Can you work these out from the model? Positions are in its coordinate system, mm. Coordinates: 2 decimals unless noted, no trailing zeros. Order: outer loops, then holes, each group sorted by start corner. A loop starts at its lowest first (then second) coordinate and runs counter-clockwise, first axis right, second up. Notation, with made-up numbers: (-11, 42.25) -> (36, 42.25) arc R28 ccw to (36, 70.25) -> close; hole circle Ø4 at (64.25, 44.25). An arc over 180 degrees is marked (long way). Return JSON: item names as keys, results as strings. Group by question number.
1) If I drill on probe 1 along Y at (x, z) = (62.5, 2.65); probe 2 along Y at (x, z) = (88.5, 0.95); probe 3 along Y at (x, z) = (99, 0.7), over which ranges is the centre line in solid material (lowest first)? Write a range as from..to.
2) If we section it at B-B, the plane y = 3755: Please give me the cut outline in (x, z), then the cut area to 3 significant figures.
3) If we section it at A-A, the plane z = 1.35: Please give me the cut outline in (x, y), then the cut area to 3 significant figures.
4) For pin 1 (11 mm diameter, centred on x = 106.6, y = 3258.06, fed in from -Z); pin 2 (23.5 mm diameter, centred on x = 86.75, y = 4138.87, fed in from -Z), each with a flat end and sliding along its axis, tell me the tip position at first contact or that it passes through.
Autodesk Inventor part; units mm, degrees
ref_plane "YZ Plane" through (0, 0, 0) normal (1, 0, 0) x (0, 1, 0)
ref_plane "XZ Plane" through (0, 0, 0) normal (0, 1, 0) x (-1, 0, 0)
ref_plane "XY Plane" through (0, 0, 0) normal (0, 0, 1) x (1, 0, 0)
sketch "Sketch1" plane through (0, 0, 0) normal (0, 0, 1) x (1, 0, 0)
  line L0 (0, 0) -> (0, 4438.8737)
  line L1 (0, 4438.8737) -> (100, 4438.8737)
  line L2 (100, 4438.8737) -> (200, 0)
  line L3 (200, 0) -> (0, 0)
  circle A0 centre (0, 0) radius 30
  line L4 (0, 1479.6246) -> (166.6667, 1479.6246)
  line L5 (0, 2959.2492) -> (133.3333, 2959.2492)
  circle A1 centre (0, 1479.6246) radius 30
  circle A2 centre (0, 2959.2492) radius 30
  line L6 (190.8761, 405) -> (120.8761, 405)
  line L7 (120.8761, 405) -> (120.8761, 410)
  line L8 (120.8761, 410) -> (190.8761, 410)
  line L9 (190.8761, 410) -> (190.8761, 405)
  line L10 (109.6148, 909.8732) -> (179.6148, 909.8732)
  line L11 (179.6148, 904.8732) -> (109.6148, 904.8732)
  line L12 (109.6148, 904.8732) -> (109.6148, 909.8732)
  line L13 (179.6148, 909.8732) -> (179.6148, 904.8732)
  line L14 (98.3535, 1409.7463) -> (168.3535, 1409.7463)
  line L15 (168.3535, 1404.7463) -> (98.3535, 1404.7463)
  line L16 (98.3535, 1404.7463) -> (98.3535, 1409.7463)
  line L17 (168.3535, 1409.7463) -> (168.3535, 1404.7463)
  line L18 (87.0923, 1909.6195) -> (157.0923, 1909.6195)
  line L19 (157.0923, 1904.6195) -> (87.0923, 1904.6195)
  line L20 (87.0923, 1904.6195) -> (87.0923, 1909.6195)
  line L21 (157.0923, 1909.6195) -> (157.0923, 1904.6195)
  line L22 (75.831, 2409.4927) -> (145.831, 2409.4927)
  line L23 (145.831, 2404.4927) -> (75.831, 2404.4927)
  line L24 (75.831, 2404.4927) -> (75.831, 2409.4927)
  line L25 (145.831, 2409.4927) -> (145.831, 2404.4927)
  line L26 (64.5698, 2909.3658) -> (134.5698, 2909.3658)
  line L27 (134.5698, 2904.3658) -> (64.5698, 2904.3658)
  line L28 (64.5698, 2904.3658) -> (64.5698, 2909.3658)
  line L29 (134.5698, 2909.3658) -> (134.5698, 2904.3658)
  line L30 (53.3085, 3409.239) -> (123.3085, 3409.239)
  line L31 (123.3085, 3404.239) -> (53.3085, 3404.239)
  line L32 (53.3085, 3404.239) -> (53.3085, 3409.239)
  line L33 (123.3085, 3409.239) -> (123.3085, 3404.239)
  line L34 (42.0472, 3909.1122) -> (112.0472, 3909.1122)
  line L35 (112.0472, 3904.1122) -> (42.0472, 3904.1122)
  line L36 (42.0472, 3904.1122) -> (42.0472, 3909.1122)
  line L37 (112.0472, 3909.1122) -> (112.0472, 3904.1122)
  line L38 (0, 1629.6246) -> (163.2874, 1629.6246)
  line L39 (0, 3079.2492) -> (130.6299, 3079.2492)
  circle A3 centre (20, 4418.8737) radius 9
  circle A4 centre (106.5967, 3258.0554) radius 9
  circle A5 centre (86.7534, 4138.8737) radius 9
  line L40 (86.7534, 4138.8737) -> (106.5967, 3258.0554)
  point P0 (30, 2959.2492)
  point P1 (0, 2929.2492)
  point P2 (0, 1509.6246)
  point P3 (0, 1449.6246)
  point P4 (0, 30)
  point P5 (30, 0)
  point P6 (190.7634, 410)
  point P7 (179.5022, 909.8732)
  point P8 (168.3535, 1404.7463)
  point P9 (168.2409, 1409.7463)
  point P10 (30, 1479.6246)
  point P11 (157.0923, 1904.6195)
  point P12 (156.9796, 1909.6195)
  point P13 (145.831, 2404.4927)
  point P14 (145.7184, 2409.4927)
  point P15 (134.5698, 2904.3658)
  point P16 (134.4571, 2909.3658)
  point P17 (0, 2989.2492)
  point P18 (123.3085, 3404.239)
  point P19 (123.1959, 3409.239)
  point P20 (112.0472, 3904.1122)
  point P21 (111.9346, 3909.1122)
  dimension "d65" = 100
  dimension "d67" = 200
  dimension "d68" = 60
  dimension "d69" = 1480
  dimension "d70" = 1480
  dimension "d71" = 1480
  dimension "d72" = 5
  dimension "d73" = 70
  dimension "d74" = 410
  dimension "d77" = 500
  dimension "d82" = 120
  dimension "d83" = 150
  dimension "d88" = 18
  dimension "d91" = 20
  dimension "d92" = 20
  dimension "d93" = 20
  dimension "d94" = 300
  dimension "d95" = 300
extrude "Plate3" add sketch "Sketch1" along normal blind 4 contours L39 L2 L5 A2 L0 | L0 L1 L2 L34 L36 L35 L40 L30 L32 L31 L39 | L30 L40 L35 L2
chamfer "Corner Chamfer2" distance 3 angle 45 4 edges at (123.3085, 3404.239, 2) (123.1959, 3409.239, 2) (112.0472, 3904.1122, 2) (111.9346, 3909.1122, 2)
equation "\"BendRadius\" = Thickness"
equation "\"BendReliefWidth\" = Thickness"
equation "\"BendReliefDepth\" = 0.5 * Thickness"
equation "\"CornerReliefSize\" = 4 * Thickness"
equation "\"MinimumRemnant\" = 2 * Thickness"
equation "\"TransitionRadius\" = BendRadius"
equation "\"JacobiRadiusSize\" = BendRadius"
equation "\"GapSize\" = Thickness"
properties part number "GBK 3311 central third rib" material "Steel"
Result sheet:
{
 "1": {"probe 1": "y = 2959.25..3404.24, 3409.24..3904.11, 3909.11..4438.87", "probe 2": "y = 2959.25..3404.24, 3409.24..3904.11, 3909.11..4130.04, 4147.7..4438.87", "probe 3": "y = 2959.25..3253.23, 3262.88..3404.24, 3409.24..3904.11, 3909.11..4438.87"},
 "2": {"outline": "(0, 0) -> (115.41, 0) -> (115.41, 4) -> (0, 4) -> close", "area": "462 mm2"},
 "3": {"outline": "(0, 2989.25) arc R30 cw to (30, 2959.25) -> (133.33, 2959.25) -> (123.38, 3401.24) -> (120.31, 3404.24) -> (53.31, 3404.24) -> (53.31, 3409.24) -> (120.2, 3409.24) -> (123.13, 3412.24) -> (112.11, 3901.11) -> (109.05, 3904.11) -> (42.05, 3904.11) -> (42.05, 3909.11) -> (108.93, 3909.11) -> (111.87, 3912.11) -> (100, 4438.87) -> (0, 4438.87) -> close; hole circle Ø18 at (20, 4418.87); hole circle Ø18 at (86.75, 4138.87); hole circle Ø18 at (106.6, 3258.06)", "area": "170,000 mm2"},
 "4": {"pin 1": "passes through", "pin 2": "stops at z = 0"}
}
